```python
from build123d import *

# Parameters (mm, degrees)
SKETCH1_R           = 1.75
BOSS_EXTRUDE1_DEPTH = 4
SKETCH2_W           = 130
SKETCH2_H           = 10.5
SKETCH2_R           = 1.75
BOSS_EXTRUDE2_DEPTH = 1
SKETCH3_R           = 1.75
BOSS_EXTRUDE3_DEPTH = 1.5
FILLET1_R           = 1


with BuildPart() as part:
    # Sketch1 → Boss-Extrude1 (new body)
    with BuildSketch(Plane(origin=(0, 0, 0), x_dir=(1, 0, 0), z_dir=(0, 1, 0))):
        with BuildLine():
            Line((-75, -8), (75, -8))
            Line((75, -8), (75, 5))
            ThreePointArc((75, 5), (74.121320344, 7.121320344), (72, 8))
            Line((72, 8), (-72, 8))
            ThreePointArc((-72, 8), (-74.121320344, 7.121320344), (-75, 5))
            Line((-75, 5), (-75, -8))
        make_face()
        with Locations(Location((-70, 0, 0), (0, 0, 270))):
            Circle(SKETCH1_R, mode=Mode.SUBTRACT)
        with BuildLine():
            ThreePointArc((61.75, 0), (61.237436867, -1.237436867), (60, -1.75))
            Line((60, -1.75), (-60, -1.75))
            ThreePointArc((-60, -1.75), (-61.75, 0), (-60, 1.75))
            Line((-60, 1.75), (60, 1.75))
            ThreePointArc((60, 1.75), (61.237436867, 1.237436867), (61.75, 0))
        make_face(mode=Mode.SUBTRACT)
        with Locations(Location((70, 0, 0), (0, 0, 270))):
            Circle(SKETCH1_R, mode=Mode.SUBTRACT)
    extrude(amount=BOSS_EXTRUDE1_DEPTH)

    # Sketch2 → Boss-Extrude2 (add)
    with BuildSketch(Plane(origin=(0, 4, 0), x_dir=(1, 0, 0), z_dir=(0, 1, 0))):
        with BuildLine():
            Line((-75, -8), (75, -8))
            Line((75, -8), (75, 5))
            ThreePointArc((75, 5), (74.121320344, 7.121320344), (72, 8))
            Line((72, 8), (-72, 8))
            ThreePointArc((-72, 8), (-74.121320344, 7.121320344), (-75, 5))
            Line((-75, 5), (-75, -8))
        make_face()
        with Locations((0, -0.75)):
            Rectangle(SKETCH2_W, SKETCH2_H, mode=Mode.SUBTRACT)
        with Locations(Location((-70, 0, 0), (0, 0, 270))):
            Circle(SKETCH2_R, mode=Mode.SUBTRACT)
        with Locations(Location((70, 0, 0), (0, 0, 270))):
            Circle(SKETCH2_R, mode=Mode.SUBTRACT)
    extrude(amount=BOSS_EXTRUDE2_DEPTH)

    # Sketch3 → Boss-Extrude3 (add)
    # profile 1 of 2: a face of its own
    with BuildSketch(Plane(origin=(0, 5, 0), x_dir=(1, 0, 0), z_dir=(0, 1, 0))):
        with BuildLine():
            Line((65, 4.5), (65, 8))
            Line((65, 8), (72, 8))
            ThreePointArc((72, 8), (74.121320344, 7.121320344), (75, 5))
            Line((75, 5), (75, -8))
            Line((75, -8), (65, -8))
            Line((65, -8), (65, -6))
            Line((65, -6), (65, 4.5))
        make_face()
        with Locations(Location((70, 0, 0), (0, 0, 270))):
            Circle(SKETCH3_R, mode=Mode.SUBTRACT)
    # profile 2 of 2: a face of its own
    with BuildSketch(Plane(origin=(0, 5, 0), x_dir=(1, 0, 0), z_dir=(0, 1, 0))):
        with BuildLine():
            Line((-65, 4.5), (-65, 8))
            Line((-65, 8), (-72, 8))
            ThreePointArc((-72, 8), (-74.121320344, 7.121320344), (-75, 5))
            Line((-75, 5), (-75, -8))
            Line((-75, -8), (-65, -8))
            Line((-65, -8), (-65, -6))
            Line((-65, -6), (-65, 4.5))
        make_face()
        with Locations(Location((-70, 0, 0), (0, 0, 270))):
            Circle(SKETCH3_R, mode=Mode.SUBTRACT)
    extrude(amount=BOSS_EXTRUDE3_DEPTH)

    # Fillet1
    fillet1_edges = [part.edges().sort_by_distance(p)[0] for p in [
        (-65, 5, 7),
        (65, 5, 7),
        (65, 5, -6.25),
        (-65, 5, -6.25),
    ]]
    fillet(fillet1_edges, radius=FILLET1_R)


solid = part.part
```
The listing builds one solid part. Answer for the finished solid, in the listing's coordinates (mm). A direction names the side the tool comes from. Give positions to 0.01 mm unless a question says otherwise; leave off trailing zeros. Write each loop counter-clockwise with the first axis right and the second up, starting at its lowest first coordinate (ties: lowest second). Pieces come first, ordered by that corner, then holes. Notation, with made-up numbers: (21, 70) -> (58, 70) arc R27 ccw to (58, 96) -> close; hole circle Ø11 at (29, 52). An arc over 180 degrees is marked (long way). Write item = value, one per line. Start each with the question number.
1) The part is cut by section C-C, the plane z = 4.75. Determine the outline of the cut face in (x, y), and give its area (3 significant figures).
2) Straight lines are drawn through the part: line 1 along Z through (x, y) = (-70, 4.5); line 2 along X through (y, z) = (1.5, 0). For each, find the intervals that lie inside material, in ascending order.
3) Which of the six approach directions +Z, -Z, +X, -X, +Y, -Y give full straight-line access (tool end or side, diameter ignored) to faces 1 (the face through (-61.75, 1.97, 0.04)), 2 (the face through (70, 6.5, -2)), 3 (the face through (-65, 5, 0))?
4) Determine the mould class of faces 4 (the face through (-1, 5, -6)), 5 (the face through (-74.1, 3.2, -7.14)), 6 (the face through (-1, 0, -2)) for opening direction X: +X half, -X half, draft (parallel to the pull), parting line (faces both ways), or undercut.
5) Each of these flat-tipped pins is pushed along its axis until it touches: pin 1 (2 mm diameter, centred on x = -10.5, z = 6.5, fed in from +Y); pin 2 (3 mm diameter, centred on x = 70, z = 0, fed in from +Y). Where does it stop, or does it pass through?
6) The part is cut by section A-A, the plane x = -70. Determine the outline of the cut face in (y, z).
7) The part is cut by section B-B, the plane y = 2.25. Determine the outline of the cut face in (x, z), and give its area (3 significant figures).
Solutions:
q1.outline = (-75, 0) -> (75, 0) -> (75, 6.5) -> (65, 6.5) -> (65, 4) -> (-65, 4) -> (-65, 6.5) -> (-75, 6.5) -> close
q1.area = 650 mm²
q2.line_1 = -8 to -1.75, 1.75 to 8
q2.line_2 = -75 to -71.75, -68.25 to -61.75, 61.75 to 68.25, 71.75 to 75
q3.face_1 = +Y, -Y
q3.face_2 = +Z, -Z, +X, -X, +Y
q3.face_3 = +Y
q4.face_4 = undercut
q4.face_5 = -X half
q4.face_6 = draft
q5.pin_1 = 5
q5.pin_2 = through
q6.outline = (0, -8) -> (6.5, -8) -> (6.5, -1.75) -> (0, -1.75) -> close; (0, 1.75) -> (6.5, 1.75) -> (6.5, 8) -> (0, 8) -> close
q7.outline = (-75, -5) arc R3 ccw to (-72, -8) -> (72, -8) arc R3 ccw to (75, -5) -> (75, 8) -> (-75, 8) -> close; hole circle Ø3.5 at (-70, 0); hole (-60, -1.75) -> (60, -1.75) arc R1.75 ccw to (60, 1.75) -> (-60, 1.75) arc R1.75 ccw to start; hole circle Ø3.5 at (70, 0)
q7.area = 1,950 mm²
